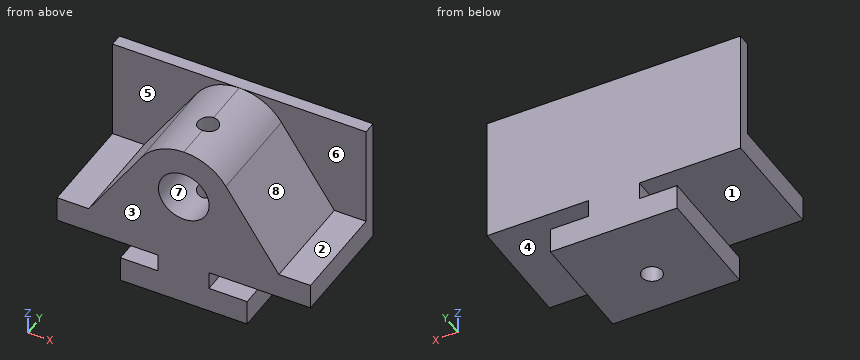
from build123d import *

# Parameters (mm, degrees)
F0_W     = 14.8242654502
F0_H     = 44.45
F0_W_2   = 95.25
F0_R     = 5.08
F0_W_3   = 16.9257345498
F1_DEPTH = 85.09
F2_R     = 12.7
F3_DEPTH = 50.8
F4_DEPTH = 50.8
F5_DEPTH = 57.151


with BuildPart() as f1:
    # F0 (on Top) → F1 (new body)
    with BuildSketch(Plane.XY):
        with Locations((-56.0878672749, 22.225)):
            Rectangle(F0_W, F0_H)
        with Locations((-1.0507345498, 22.225)):
            Rectangle(F0_W_2, F0_H)
        with Locations((0, 22.225)):
            Circle(F0_R, mode=Mode.SUBTRACT)
        Polygon((-63.5, 57.15), (-63.5, 44.45), (-48.6757345498, 44.45), (46.5742654502, 44.45), (63.5, 44.45), (63.5, 57.15), align=None)
        with Locations((55.0371327251, 22.225)):
            Rectangle(F0_W_3, F0_H)
    extrude(amount=F1_DEPTH)

    # F2 (on face) → F3 (cut)
    with BuildSketch(Plane.XZ):
        with Locations((0, 59.69)):
            Circle(F2_R)
    extrude(amount=-F3_DEPTH, mode=Mode.SUBTRACT)

    # F2 (on face) → F4 (cut)
    with BuildSketch(Plane.XZ):
        with BuildLine():
            Line((-63.5, 85.09), (-63.5, 34.29))
            Line((-63.5, 34.29), (-47.625, 34.29))
            Line((-47.625, 34.29), (-21.0934256055, 73.8401730104))
            ThreePointArc((-21.0934256055, 73.8401730104), (-11.9529410666, 82.1017647645), (2.49e-07, 85.09))
            Line((2.49e-07, 85.09), (-63.5, 85.09))
        make_face()
        with BuildLine():
            Line((47.625, 34.29), (63.5, 34.29))
            Line((63.5, 34.29), (63.5, 85.09))
            Line((63.5, 85.09), (2.49e-07, 85.09))
            ThreePointArc((2.49e-07, 85.09), (11.9529412863, 82.1017646473), (21.0934256055, 73.8401730104))
            Line((21.0934256055, 73.8401730104), (47.625, 34.29))
        make_face()
    extrude(amount=-F4_DEPTH, mode=Mode.SUBTRACT)

    # F2 (on face) → F5 (cut, through all)
    with BuildSketch(Plane.XZ):
        Polygon((-63.5, 0), (-31.75, 0), (-31.75, 12.7), (-12.8072916996, 12.7), (-12.8072916996, 21.59), (-63.5, 21.59), align=None)
        Polygon((31.75, 12.7), (31.75, 0), (63.5, 0), (63.5, 21.59), (12.5927083004, 21.59), (12.5927083004, 12.7), align=None)
    extrude(amount=-F5_DEPTH, mode=Mode.SUBTRACT)


solid = f1.part
Model file for the job. Use its own axes, mm. Face numbers are marked on the shaded views. A direction names the side the tool comes from. Coordinates: 2 decimals unless noted, no trailing zeros. Write each loop counter-clockwise with the first axis right and the second up, starting at its lowest first coordinate (ties: lowest second). Pieces come first, ordered by that corner, then holes. Notation, with made-up numbers: (12, 60.25) - (32, 60.25) arc R20 cw to (32, 89.25) - close; hole circle Ø5 at (83.25, -20). An arc over 180 degrees is marked (long way). Write each question's results on one line, items separated by ' | '. Start each with the question number.
1) Cut at B-B (x = 27). Write the cut outline in (y, z).
2) Cut at C-C (z = 36). Write the cut outline in (x, y) (3 decimals), then the cut area to 3 significant figures.
3) Cut at A-A (y = 3). Write the cut outline in (x, z) (3 decimals), then the cut area to 3 significant figures.
4) 3-axis set-ups, long thin cutter, end or side, ignore diameter. For the marked faces 1, 2, 3, 4 and 5: which of +Z, -Z, +X, -X, +Y, -Y reach the whole face in a straight line?
5) Flat gauge pins, fed straight in: P1, Ø12.5, axis at x = -2, z = 61.5, coming from the -Y side; P2, Ø3, axis at y = 24.5, z = 35, coming from the +X side; P3, Ø1.5, axis at y = 45, z = 68.5, coming from the +X side; P4, Ø4, axis at y = 24.5, z = 7, coming from the -X side. Where does each tip first touch, or does it go through?
6) Probe line 1 along Y through (x, z) = (0, 23) (3 decimals); line 2 along Z through (x, y) = (53.5, 14); line 3 along Y through (x, z) = (41.5, 77). List the from-to ranges inside material, lowest first. Write a range as from..to.
7) Mould opens along Z. For the marked faces 6, 7 and 8 say: pulls with the +Z half, pulls with the -Z half, needs draft (parallel to the pull), parting line crosses it, or undercut.
Returned:
1) outline: (0, 0) - (57.15, 0) - (57.15, 12.7) - (0, 12.7) - close; (0, 21.59) - (57.15, 21.59) - (57.15, 85.09) - (50.8, 85.09) - (50.8, 65.04) - (0, 65.04) - close
2) outline: (-63.5, 50.8) - (-46.478, 50.8) - (-46.478, 0) - (46.478, 0) - (46.478, 50.8) - (63.5, 50.8) - (63.5, 57.15) - (-63.5, 57.15) - close; hole circle Ø10.16 at (0, 22.225) | area: 5,450 mm^2
3) outline: (-63.5, 21.59) - (-12.807, 21.59) - (-12.807, 12.7) - (-31.75, 12.7) - (-31.75, 0) - (31.75, 0) - (31.75, 12.7) - (12.593, 12.7) - (12.593, 21.59) - (63.5, 21.59) - (63.5, 34.29) - (47.625, 34.29) - (21.093, 73.84) arc R25.4 ccw to (-21.093, 73.84) - (-47.625, 34.29) - (-63.5, 34.29) - close; hole circle Ø25.4 at (0, 59.69) | area: 5,190 mm^2
4) face 1: -X, +Y, -Y | face 2: +Z, +X, -Y | face 3: +Z, -Z, +X, -X, -Y | face 4: +X, +Y, -Y | face 5: +Z, -X, -Y
5) P1: y = 50.8 | P2: x = 63.5 | P3: x = 25.18 | P4: x = -31.75
6) line 1: 0..17.145, 27.305..57.15 | line 2: 21.59..34.29 | line 3: 50.8..57.15
7) face 6: needs draft | face 7: undercut | face 8: pulls with the +Z half
